Model file for the job. Use its own axes, mm. Give positions to 0.01 mm unless a question says otherwise; leave off trailing zeros. Loops run counter-clockwise (first coordinate to the right, second up) from the corner with the lowest first, then second, coordinate; pieces in that order, holes last. Notation, with made-up numbers: M 5.5,44.5 L 27.5,44.5 A15 cw 27.5,63.5 Z; hole C 79,-6.75 d6. An arc over 180 degrees is marked long. Use CSV: the item, a comma, the result in double quotes. Start each with the question number.
(1) Slice it at A-A on x = 0. State how many separate pieces and enclosed holes the cut face has, and give its area (3 significant figures).
(2) Slice it at D-D on y = 18. List the corners of the cut face in (x, z).
(3) Slice it at B-B on z = 1.4. List the corners of the cut face in (x, y) (1 decimal).
(4) Two-plate mould, pull along Y, no slides. Class faces 1 (the face through (43.124, -13.58, 2.348)), 2 (the face through (-1, 1, 0)), 3 (the face through (-0.344, -44.412, 2.415)): pulls with the +Y half, pulls with the -Y half, needs draft (parallel to the pull), parting line crosses it, or undercut.
(5) Slice it at C-C on x = 37.12. List the corners of the cut face in (y, z), and give its area (3 significant figures).
(6) Flat gauge pins, fed straight in: P1, Ø2.5, axis at x = 0, y = -42.86, coming from the -Z side; P2, Ø2, axis at x = 20, z = 4, coming from the -Y side. Where does each tip first touch, or does it go through?
(7) Wall check: line 1 along Y through (x, z) = (0, 3.8) (3 decimals); line 2 along Y through (x, z) = (-37.12, 2.9); line 3 along X through (y, z) = (21.5, 2.55). Give the ranges that are in metal, low to high. Write a range as from..to.
Autodesk Inventor part; units mm, degrees
ref_plane "YZ Plane" through (0, 0, 0) normal (1, 0, 0) x (0, 1, 0)
ref_plane "XZ Plane" through (0, 0, 0) normal (0, 1, 0) x (-1, 0, 0)
ref_plane "XY Plane" through (0, 0, 0) normal (0, 0, 1) x (1, 0, 0)
sketch "Sketch1" plane through (0, 0, 0) normal (0, 0, 1) x (1, 0, 0)
  circle A0 centre (0, 0) radius 45.212
  dimension "d0" = 90.424
extrude "Extrusion1" add sketch "Sketch1" along normal blind 4.7625
sketch "Sketch4" plane through (0, 0, 4.7625) normal (0, 0, 1) x (1, 0, 0)
  circle A0 centre (0, 42.8625) radius 1.5875
  circle A1 centre (-37.12, 21.4313) radius 1.5875
  circle A2 centre (-37.12, -21.4312) radius 1.5875
  circle A3 centre (0, -42.8625) radius 1.5875
  circle A4 centre (37.12, -21.4313) radius 1.5875
  circle A5 centre (37.12, 21.4312) radius 1.5875
  point P0 (0, 0)
  dimension "d14" = 3.175
  dimension "d15" = 42.8625
  dimension "d18" = 360
extrude "Extrusion4" cut sketch "Sketch4" against normal blind 25.4
properties part number "AluminumSealingDiscMidshipsMiddle" material "Aluminum 6061"
Reply:
1,separate pieces,"3"
1,enclosed holes,"0"
1,area,"400 mm^2"
2,outline,"M -41.47,0 L 41.47,0 L 41.47,4.76 L -41.47,4.76 Z"
3,outline,"C 0,0 d90.4; hole C -37.1,-21.4 d3.2; hole C -37.1,21.4 d3.2; hole C 0,-42.9 d3.2; hole C 0,42.9 d3.2; hole C 37.1,-21.4 d3.2; hole C 37.1,21.4 d3.2"
4,face 1,"parting line crosses it"
4,face 2,"needs draft"
4,face 3,"undercut"
5,outline,"M -25.81,0 L -23.02,0 L -23.02,4.76 L -25.81,4.76 Z; M -19.84,0 L 19.84,0 L 19.84,4.76 L -19.84,4.76 Z; M 23.02,0 L 25.81,0 L 25.81,4.76 L 23.02,4.76 Z"
5,area,"216 mm^2"
6,P1,"passes through"
6,P2,"stops at y = -41.03"
7,line 1,"y = -45.212..-44.45, -41.275..41.275, 44.45..45.212"
7,line 2,"y = -25.81..-23.02, -19.84..19.84, 23.02..25.81"
7,line 3,"x = -39.77..-38.71, -35.53..35.53, 38.71..39.77"
